Here's the drawing with two shaded views (mm, measured from the low corner). I have some questions. A direction names the side the tool comes from. Round coordinates to 2 decimals unless told otherwise and drop trailing zeros. Order: outer loops, then holes, each group sorted by start corner. A loop starts at its lowest first (then second) coordinate and runs counter-clockwise, first axis right, second up. Notation, with made-up numbers: (85, -24.5) -> (111, -24.5) arc R15 ccw to (111, -17.5) -> close; hole circle Ø3 at (37.5, 44.25). An arc over 180 degrees is marked (long way). One line per question, with ' | ' between items.
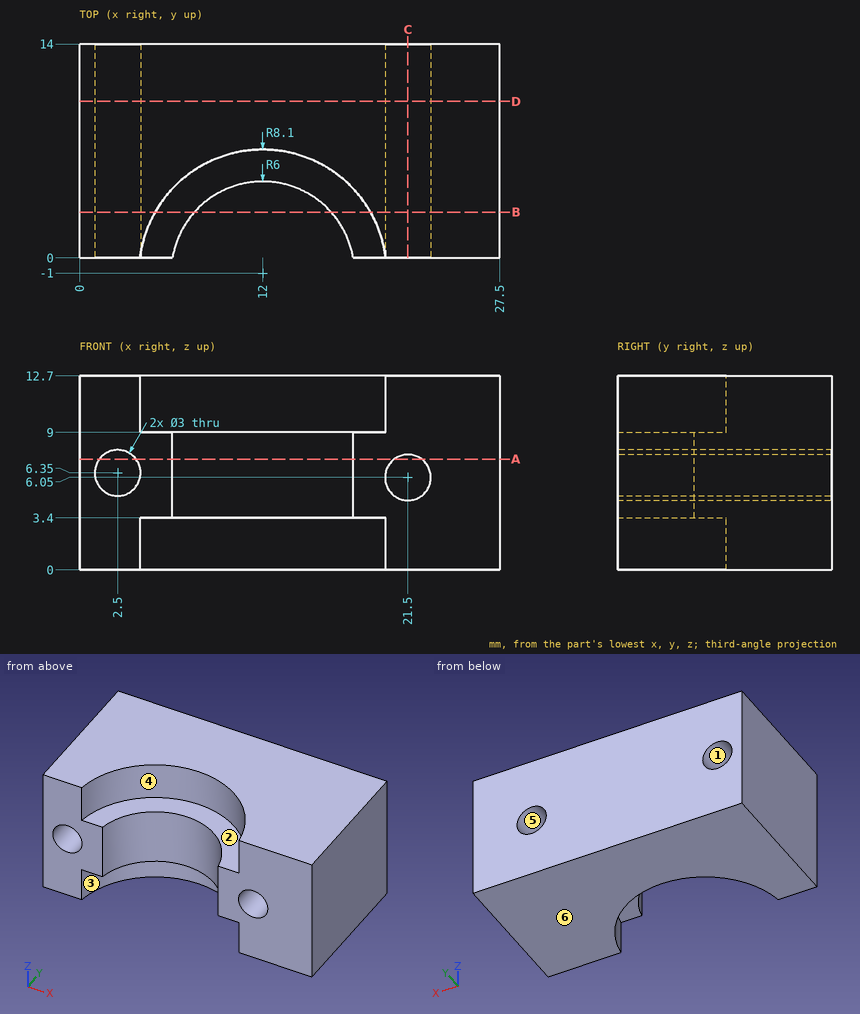
1. On a 3-axis mill with a long thin cutter (end or side, diameter ignored), from which of +Z, -Z, +X, -X, +Y, -Y can I reach the whole of each face in a straight line? I mean the marked faces 1, 2 and 3. Say none if no direction works.
From the geometry:
face 1: +Y, -Y | face 2: +Z, -Y | face 3: -Z, -Y
2. I want a section at A-A on z = 7.25. List the corners of the cut face in (x, y) for me, and give its area (3 significant figures).
From the geometry:
outline: (0, 0) -> (1.3, 0) -> (1.3, 14) -> (0, 14) -> close; (3.7, 0) -> (6.08, 0) arc R6 cw to (17.92, 0) -> (20.6, 0) -> (20.6, 14) -> (3.7, 14) -> close; (22.4, 0) -> (27.5, 0) -> (27.5, 14) -> (22.4, 14) -> close | area: 282 mm²
3. I want a section at B-B on y = 3. List the corners of the cut face in (x, z) for me.
From the geometry:
outline: (0, 0) -> (4.96, 0) -> (4.96, 3.4) -> (7.53, 3.4) -> (7.53, 9) -> (4.96, 9) -> (4.96, 12.7) -> (0, 12.7) -> close; (16.47, 3.4) -> (19.04, 3.4) -> (19.04, 0) -> (27.5, 0) -> (27.5, 12.7) -> (19.04, 12.7) -> (19.04, 9) -> (16.47, 9) -> close; hole circle Ø3 at (2.5, 6.35); hole circle Ø3 at (21.5, 6.05)
4. I need wall thicknesses on probe 1 along X at (y, z) = (5.5, 6.35); probe 2 along Z at (x, y) = (11.25, 6.25); probe 3 along Z at (x, y) = (21, 6). Which ranges of each line are inside material? Lowest first, please.
From the geometry:
probe 1: x = 0 to 1, 4 to 20.03, 22.97 to 27.5 | probe 2: z = 3.4 to 9 | probe 3: z = 0 to 4.64, 7.46 to 12.7
5. I want a section at C-C on x = 21.5. List the corners of the cut face in (y, z) for me.
From the geometry:
outline: (0, 0) -> (14, 0) -> (14, 4.55) -> (0, 4.55) -> close; (0, 7.55) -> (14, 7.55) -> (14, 12.7) -> (0, 12.7) -> close
6. I want a section at D-D on y = 10.25. List the corners of the cut face in (x, z) for me.
From the geometry:
outline: (0, 0) -> (27.5, 0) -> (27.5, 12.7) -> (0, 12.7) -> close; hole circle Ø3 at (2.5, 6.35); hole circle Ø3 at (21.5, 6.05)
7. If we mould it in two halves opening along Z, with no side actions, what happens to the marked faces 4, 5 and 6? For each: pulls with the +Z half, pulls with the -Z half, needs draft (parallel to the pull), parting line crosses it, or undercut.
From the geometry:
face 4: needs draft | face 5: undercut | face 6: pulls with the -Z half
8. I'm going to push a flat-ended pin straight in: pin 1 (3.5 mm diameter, centred on x = 11.5, y = 5, fed in from +Z). Where does the tip first touch, or does it pass through?
From the geometry:
pin 1: stops at z = 9
